Design review of the part built by this model. Coordinates are the model's own, in mm. A direction names the side the tool comes from. Coordinates: 2 decimals unless noted, no trailing zeros. Write each loop counter-clockwise with the first axis right and the second up, starting at its lowest first coordinate (ties: lowest second). Pieces come first, ordered by that corner, then holes.
Q1. Take a section at B-B (y = -1.75). Give the boundary of the cut face in (x, z), and give its area (3 significant figures).
Q2. Machinability: for faces 5 (the flat face through (0, -6.3, -4)), 6 (the flat face through (5, -3, -2)), which of the approach directions +Z, -Z, +X, -X, +Y, -Y give a long, thin tool a straight path to every point of the face, cutting with its end or side? Answer none if there is none.
Q3. Take a section at D-D (x = -2). Give the boundary of the cut face in (y, z).
Q4. Take a section at A-A (z = 0). Give the boundary of the cut face in (x, y), and give its area (3 significant figures).
Q5. Take a section at C-C (x = -0.75). Give the boundary of the cut face in (y, z).
Q6. Mouldability with a two-part tool opening along Z and no side actions: class faces 1 (the cylindrical face through (3.233, -7.459, -1.341)), 2 (the flat face through (4.85, -3, 0)), 3 (the flat face through (-5, -3, 0)), 4 (the flat face through (2.535, -3.106, 4.31)) as pulls with the +Z half, pulls with the -Z half, needs draft (parallel to the pull), parting line crosses it, or undercut.
Q7. Insertion check: pin 1 (4 mm diameter, centred on x = -4, y = -3.5, fed in from +Z). The pin has a flat end and moves straight along its axis. Give the tip position at first contact, or say it passes through.
Q8. For probe 1 along Y at (x, z) = (3.5, -3.5); probe 2 along Z at (x, y) = (0.79, -6); probe 3 along Z at (x, y) = (-0.75, -1.25), list the stretches that pass through material, from the lowest coordinate up.
```python
from build123d import *

# Parameters (mm, degrees)
F0_R     = 2.5
F1_DEPTH = 6.3
F3_R     = 3.5
F4_DEPTH = 2.35
F5_DEPTH = 8.65
F0_W     = 0.15
F0_H     = 2
F8_DEPTH = 22


# Not quite as in the source:
# - an extrude ends at something that could not be found from the text; its depth is read off the source's solid
# - a feature names something its author has since deleted; it is built from what else it names


with BuildPart() as f1:
    # F0 (on Front) → F1 (new body)
    with BuildSketch(Plane.XZ):
        Polygon((5, 1), (5, 2.8867513459), (0, 5.7735026919), (-5, 2.8867513459), (-5, -2.8867513459), (0, -5.7735026919), (5, -2.8867513459), (5, -1), (4.85, -1), (4.85, 1), align=None)
        with Locations((0.79, 0)):
            Circle(F0_R, mode=Mode.SUBTRACT)
    extrude(amount=F1_DEPTH)

    # F3 (on offset) → F4 (join)
    with BuildSketch(Plane.XZ.offset(6.3)):
        Circle(F3_R)
    extrude(amount=F4_DEPTH)

    # F0 (on Front) → F5 (cut, through all)
    with BuildSketch(Plane.XZ):
        with Locations((0.79, 0)):
            Circle(F0_R)
    extrude(amount=F5_DEPTH, mode=Mode.SUBTRACT)

    # F6 (on Top) → F7 (revolve, cut)
    with BuildSketch(Plane.XY):
        Polygon((-6.0966597098, -6.5938490836), (-5, -6.3), (-6.0966597098, -6.3), align=None)
    revolve(axis=Axis((0, -6.5372320823, 0), (0, -1, 0)), mode=Mode.SUBTRACT)

    # F0 (on Front) → F8 (cut, through all)
    with BuildSketch(Plane.XZ):
        with Locations((4.925, 0)):
            Rectangle(F0_W, F0_H)
    extrude(amount=-F8_DEPTH, mode=Mode.SUBTRACT)


solid = f1.part
```
Response:
1. outline: (-5, -2.89) - (0, -5.77) - (5, -2.89) - (5, -1) - (4.85, -1) - (4.85, 1) - (5, 1) - (5, 2.89) - (0, 5.77) - (-5, 2.89) - close; hole circle Ø5 at (0.79, 0)
1. area: 66.7 mm2
2. face 5: -Y
2. face 6: +Z, -Z, +X, +Y, -Y
3. outline: (-8.65, -2.87) - (-6.3, -2.87) - (-6.3, -4.62) - (0, -4.62) - (0, 4.62) - (-6.3, 4.62) - (-6.3, 2.87) - (-8.65, 2.87) - close
4. outline: (-5, -6.3) - (-3.5, -6.3) - (-3.5, -8.65) - (-1.71, -8.65) - (-1.71, 0) - (-5, 0) - close; (3.29, -8.65) - (3.5, -8.65) - (3.5, -6.3) - (4.85, -6.3) - (4.85, 0) - (3.29, 0) - close
4. area: 35.3 mm2
5. outline: (-8.65, -3.42) - (-6.3, -3.42) - (-6.3, -5.34) - (0, -5.34) - (0, -1.97) - (-8.65, -1.97) - close; (-8.65, 1.97) - (0, 1.97) - (0, 5.34) - (-6.3, 5.34) - (-6.3, 3.42) - (-8.65, 3.42) - close
6. face 1: parting line crosses it
6. face 2: undercut
6. face 3: needs draft
6. face 4: pulls with the +Z half
7. pin 1: stops at z = 4.62
8. probe 1: y = -6.3 to 0
8. probe 2: z = -5.32 to -2.5, 2.5 to 5.32
8. probe 3: z = -5.34 to -1.97, 1.97 to 5.34
